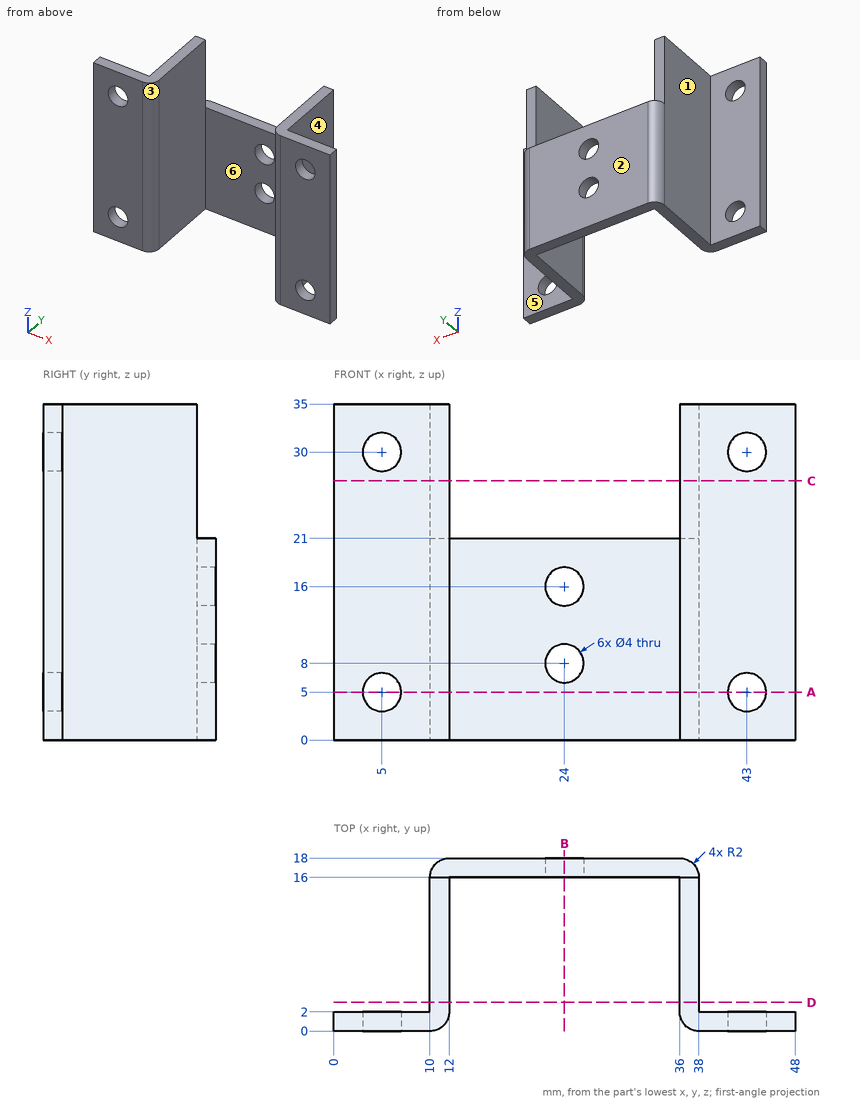
The figure shows three views and two pictorial views of one solid part (mm, origin at its lowest corner). Answer the questions. A direction names the side the tool comes from. Give positions to 0.01 mm unless a question says otherwise; leave off trailing zeros. Write each loop counter-clockwise with the first axis right and the second up, starting at its lowest first coordinate (ties: lowest second). Pieces come first, ordered by that corner, then holes. Notation, with made-up numbers: (-33.75, 77.25) - (10.25, 77.25) arc R22 ccw to (10.25, 96.25) - close; hole circle Ø7 at (-4.5, -29.75). An arc over 180 degrees is marked (long way). Use one line per item in the form item = value. Start each with the question number.
1) Find section A-A on z = 5. Determine the outline of the cut face in (x, y), plus the area to 3 significant figures.
2) Find section B-B on x = 24. Determine the outline of the cut face in (y, z).
3) A tool of negligible diameter and unlimited length cuts with its end or side. For the marked faces 1, 2 and 3, from which of +Z, -Z, +X, -X, +Y, -Y can it reach the whole face along a straight path? Write none if from no direction.
4) The mould has two halves that part along X. Classify the marked faces 4, 5 and 6: pulls with the +X half, pulls with the -X half, needs draft (parallel to the pull), parting line crosses it, or undercut.
5) Flat-ended cylindrical pins translate along their axes: pin 1 Ø4 at (y, z) = (10.5, 23) entering from -X; pin 2 Ø1 at (x, y) = (19.5, 17.5) entering from +Z; pin 3 Ø8 at (x, z) = (6.5, 25) entering from +Y. Find the tip coordinate at first contact, or state that the pin passes through.
6) Consider line 1 along Z through (x, y) = (43, 0.65); line 2 along X through (y, z) = (9, 33); line 3 along Z through (x, y) = (24, 17.2). Determine where each line is inside the solid, lowest interval first. Write a range as from..to.
7) Find section D-D on y = 3. Determine the outline of the cut face in (x, z), plus the area to 3 significant figures.
8) Find section C-C on z = 27. Determine the outline of the cut face in (x, y), plus the area to 3 significant figures.
Geometry results:
q1.outline = (0, 0) - (3, 0) - (3, 2) - (0, 2) - close; (7, 0) - (10, 0) arc R2 ccw to (12, 2) - (12, 16) - (36, 16) - (36, 2) arc R2 ccw to (38, 0) - (41, 0) - (41, 2) - (38, 2) - (38, 16) arc R2 ccw to (36, 18) - (12, 18) arc R2 ccw to (10, 16) - (10, 2) - (7, 2) - close; (45, 0) - (48, 0) - (48, 2) - (45, 2) - close
q1.area = 141 mm2
q2.outline = (16, 0) - (18, 0) - (18, 6) - (16, 6) - close; (16, 10) - (18, 10) - (18, 14) - (16, 14) - close; (16, 18) - (18, 18) - (18, 21) - (16, 21) - close
q3.face_1 = +Z, -Z, -X, +Y
q3.face_2 = +Z, -Z, +X, -X, +Y
q3.face_3 = +Z, -Z, -Y
q4.face_4 = pulls with the +X half
q4.face_5 = needs draft
q4.face_6 = undercut
q5.pin_1 = 10
q5.pin_2 = 21
q5.pin_3 = 16
q6.line_1 = 0..3, 7..28, 32..35
q6.line_2 = 10..12, 36..38
q6.line_3 = 0..6, 10..14, 18..21
q7.outline = (10, 0) - (12, 0) - (12, 35) - (10, 35) - close; (36, 0) - (38, 0) - (38, 35) - (36, 35) - close
q7.area = 140 mm2
q8.outline = (0, 0) - (10, 0) arc R2 ccw to (12, 2) - (12, 16) - (10, 16) - (10, 2) - (0, 2) - close; (36, 2) arc R2 ccw to (38, 0) - (48, 0) - (48, 2) - (38, 2) - (38, 16) - (36, 16) - close
q8.area = 102 mm2
